from build123d import *

# Parameters (mm, degrees)
F1_DEPTH = 75


with BuildPart() as f1:
    # F0 (on Front) → F1 (new body)
    with BuildSketch(Plane.XZ):
        with BuildLine():
            Line((22, 3.879194), (0, 0))
            Line((0, 0), (-5.209445, 29.544233))
            Line((-5.209445, 29.544233), (-9.148676, 28.84964))
            Line((-9.148676, 28.84964), (-7.319728, 18.477157))
            ThreePointArc((-7.319728, 18.477157), (-8.209606, 10.190581), (-13.385038, 3.658036))
            Line((-13.385038, 3.658036), (-22.725306, -3))
            Line((-22.725306, -3), (27.274694, -3))
            Line((27.274694, -3), (22.466267, 24.269941))
            Line((22.466267, 24.269941), (18.527036, 23.575349))
            Line((18.527036, 23.575349), (22, 3.879194))
        make_face()
    extrude(amount=F1_DEPTH)


solid = f1.part
Design review of the part built by this model. Coordinates are the model's own, in mm. A direction names the side the tool comes from. Give positions to 0.01 mm unless a question says otherwise; leave off trailing zeros. Order: outer loops, then holes, each group sorted by start corner. A loop starts at its lowest first (then second) coordinate and runs counter-clockwise, first axis right, second up. Notation, with made-up numbers: (11.25, -39.5) - (15.25, -39.5) arc R12 ccw to (15.25, -34.5) - close; hole circle Ø4 at (60, 20.25). An arc over 180 degrees is marked (long way). Use CSV: the item, a comma, the result in double quotes. Start each with the question number.
Q1. Take a section at C-C (y = -26.5). State the section outline as (x, z) points, and give its area (3 significant figures).
Q2. Machinability: for faces 1 (the face through (-2.57, -36.98, 14.57)), 2 (the face through (20.24, -36.98, 13.87)), 3 (the face through (-2, -75, 7)), which of the approach directions +Z, -Z, +X, -X, +Y, -Y give a long, thin tool a straight path to every point of the face, cutting with its end or side? Answer none if there is none.
Q3. Take a section at B-B (x = 19.5). State the section outline as (y, z) points.
Q4. Take a section at A-A (z = 11). State the section outline as (x, y) points.
Q5. Draft analysis for pull direction X (two halves, no side actions). For faces 4 (the face through (-8.247, -36.975, 23.736)), 5 (the face through (24.904, -36.975, 10.444)), 6 (the face through (20.524, -36.975, 23.928)), state which applies: pulls with the +X half, pulls with the -X half, needs draft (parallel to the pull), parting line crosses it, or undercut.
Q6. Take a section at D-D (x = 1.5). State the section outline as (y, z) points, and give its area (3 significant figures).
Q7. For line 1 (X direction, y = -29.5, z = 18); line 2 (X direction, y = -41.5, z = 19.5); line 3 (Z direction, x = -18.5, y = -30), list the stretches that pass through material, from the lowest coordinate up.
Q8. For P1, Ø1.5, axis at y = -60, z = 4, coming from the -X side; P2, Ø10, axis at y = -22.5, z = 12, coming from the -X side; P3, Ø1.5, axis at x = 5.5, y = -15, coming from the +Z side, all flat-tipped, find the tip position at first contact; note any pin that passes through.
Calculated:
1,outline,"(-22.73, -3) - (27.27, -3) - (22.47, 24.27) - (18.53, 23.58) - (22, 3.88) - (0, 0) - (-5.21, 29.54) - (-9.15, 28.85) - (-7.32, 18.48) arc R15 cw to (-13.39, 3.66) - close"
1,area,"484 mm²"
2,face 1,"+Z, +Y, -Y"
2,face 2,"+Y, -Y"
2,face 3,"+Z, -Z, +X, -X, -Y"
3,outline,"(-75, -3) - (0, -3) - (0, 3.44) - (-75, 3.44) - close; (-75, 18.06) - (0, 18.06) - (0, 23.75) - (-75, 23.75) - close"
4,outline,"(-7.91, -75) - (-1.94, -75) - (-1.94, 0) - (-7.91, 0) - close; (20.74, -75) - (24.81, -75) - (24.81, 0) - (20.74, 0) - close"
5,face 4,"pulls with the -X half"
5,face 5,"pulls with the +X half"
5,face 6,"undercut"
6,outline,"(-75, -3) - (0, -3) - (0, 0.26) - (-75, 0.26) - close"
6,area,"245 mm²"
7,line 1,"x = -7.24 to -3.17, 19.51 to 23.57"
7,line 2,"x = -7.5 to -3.44, 19.25 to 23.31"
7,line 3,"z = -3 to 0.01"
8,P1,"stops at x = -13.96"
8,P2,"stops at x = -10"
8,P3,"stops at z = 1.1"
